Source: CAD feature listing. Evaluate the final solid. Frame: model axes, mm. A direction names the side the tool comes from. Round coordinates to 2 decimals unless told otherwise and drop trailing zeros. Loops run counter-clockwise (first coordinate to the right, second up) from the corner with the lowest first, then second, coordinate; pieces in that order, holes last. Notation, with made-up numbers: (12.25, 5) -> (42.25, 5) arc R17 cw to (42.25, 28) -> close; hole circle Ø11 at (-1.75, 54.5). An arc over 180 degrees is marked (long way). Put each result on its own line as item: value. Start each with the question number.
1. Draft query along Y for faces 1 (the flat face through (166, 155, 9)), 2 (the flat face through (160, 160, 5)), 3 (the flat face through (175.518, 154.305, 4.93)). Return one class per face: pulls with the +Y half, pulls with the -Y half, needs draft (parallel to the pull), parting line crosses it, or undercut.
2. Cut plane A-A (z = 4.25). Return the cut outline in (x, y).
3. Cut plane C-C (y = 115). Return the cut outline in (x, z).
4. Set-up query: faces 4 (the flat face through (161.065, 159.651, 4.944)), 5 (the flat face through (330.5, 320.04, 9.37)). Return all of +Z, -Z, +X, -X, +Y, -Y with unobstructed straight access to the full face (end or side cutting, diameter ignored); none if empty.
5. Cut plane B-B (x = 281). Return the cut outline in (y, z).
6. Contact query for flat-ended pins moving along their axis: pin 1 (4 mm diameter, centred on x = 12.37, y = 1.77, fed in from +Z); pin 2 (2 mm diameter, centred on y = 97.5, z = 8.5, fed in from +X); pin 3 (1.5 mm diameter, centred on x = 56, z = 3.5, fed in from -Y). Output: stop coordinate, or through.
7. Material intervals for L1, parallel to Z at x = 82, y = 70.5; L2, parallel to X at y = 269.5, z = 6.5; L3, parallel to Y at x = 286, z = 7.75, sorted ascending.
```python
from build123d import *

# Parameters (mm, degrees)
SKETCH_1_R          = 1.6
EXTRUDE_1_DEPTH     = 10
SKETCH_2_W          = 8
SKETCH_2_H          = 13
CUT_EXTRUDE_1_DEPTH = 1000


with BuildPart() as part:
    # ｽｹｯﾁ1 → ﾎﾞｽ - 押し出し1 (new body)
    with BuildSketch(Plane.XY):
        Polygon((325.269119346, 325.269119346), (335.875721064, 314.662517628), (10.606601718, -10.606601718), (0, 0), align=None)
        with Locations((100.519119346, 89.912517628)):
            Circle(SKETCH_1_R, mode=Mode.SUBTRACT)
        with Locations((12.374368671, 1.767766953)):
            Circle(SKETCH_1_R, mode=Mode.SUBTRACT)
        with Locations((325.269119346, 314.662517628)):
            Circle(SKETCH_1_R, mode=Mode.SUBTRACT)
    extrude(amount=EXTRUDE_1_DEPTH)

    # ｽｹｯﾁ2 → ｶｯﾄ - 押し出し1 (cut)
    with BuildSketch(Plane(origin=(0, 0, 0), x_dir=(0, 0, 1), z_dir=(-0.7071067811865517, -0.7071067811865435, 0))):
        with Locations((5, -7.5)):
            Rectangle(SKETCH_2_W, SKETCH_2_H)
    extrude(amount=-CUT_EXTRUDE_1_DEPTH, mode=Mode.SUBTRACT)


solid = part.part
```
Solution:
1. face 1: undercut
1. face 2: pulls with the +Y half
1. face 3: pulls with the -Y half
2. outline: (0, 0) -> (0.71, -0.71) -> (325.98, 324.56) -> (325.27, 325.27) -> close; (9.9, -9.9) -> (10.61, -10.61) -> (335.88, 314.66) -> (335.17, 315.37) -> close
3. outline: (115, 0) -> (136.21, 0) -> (136.21, 10) -> (115, 10) -> close; hole (116.41, 1) -> (134.8, 1) -> (134.8, 9) -> (116.41, 9) -> close
4. face 4: none
4. face 5: +Z, -Z, +X, +Y
5. outline: (259.79, 0) -> (281, 0) -> (281, 10) -> (259.79, 10) -> close; hole (261.2, 1) -> (279.59, 1) -> (279.59, 9) -> (261.2, 9) -> close
6. pin 1: stops at z = 10
6. pin 2: stops at x = 119.71
6. pin 3: stops at y = 34.04
7. L1: z = 0 to 1, 9 to 10
7. L2: x = 269.5 to 270.91, 289.3 to 290.71
7. L3: y = 264.79 to 266.2, 284.59 to 286
